from build123d import *

# Parameters (mm, degrees)
SCHIZZO1_R                   = 3.85
SCHIZZO1_R_2                 = 2.35
ESTRUSIONE_ESTRUSIONE1_DEPTH = 4
ESTRUSIONE_ESTRUSIONE2_DEPTH = 1.5
TAGLIO_ESTRUSIONE1_REACH     = 18.501
SCHIZZO4_R                   = 0.5


with BuildPart() as part:
    # Schizzo1 → Estrusione-Estrusione1 (new body)
    with BuildSketch(Plane.XY):
        Circle(SCHIZZO1_R)
        Circle(SCHIZZO1_R_2, mode=Mode.SUBTRACT)
    extrude(amount=ESTRUSIONE_ESTRUSIONE1_DEPTH)

    # Schizzo3 → Estrusione-Estrusione2 (add)
    with BuildSketch(Plane(origin=(0, 0, 0), x_dir=(-1, 0, 0), z_dir=(0, 0, -1))):
        with BuildLine():
            Line((0, 3.1), (13.85, 2))
            ThreePointArc((13.85, 2), (15.85, 0), (13.85, -2))
            Line((13.85, -2), (0, -3.1))
            ThreePointArc((0, -3.1), (-3.1, 0), (0, 3.1))
        make_face()
    extrude(amount=-ESTRUSIONE_ESTRUSIONE2_DEPTH)

    # Schizzo4 → Taglio-Estrusione1 (cut, up to next)
    with BuildSketch(Plane.XY.offset(1.5), mode=Mode.PRIVATE) as taglio_estrusione1_sk1:
        with Locations((-4.85, 0)):
            Circle(SCHIZZO4_R)
    taglio_estrusione1_tool1 = extrude(taglio_estrusione1_sk1.sketch, amount=-TAGLIO_ESTRUSIONE1_REACH, mode=Mode.PRIVATE) & part.part
    # Schizzo4 → Taglio-Estrusione1 (cut, up to next)
    with BuildSketch(Plane.XY.offset(1.5), mode=Mode.PRIVATE) as taglio_estrusione1_sk2:
        with Locations((-6.85, 0)):
            Circle(SCHIZZO4_R)
    taglio_estrusione1_tool2 = extrude(taglio_estrusione1_sk2.sketch, amount=-TAGLIO_ESTRUSIONE1_REACH, mode=Mode.PRIVATE) & part.part
    # Schizzo4 → Taglio-Estrusione1 (cut, up to next)
    with BuildSketch(Plane.XY.offset(1.5), mode=Mode.PRIVATE) as taglio_estrusione1_sk3:
        with Locations((-8.85, 0)):
            Circle(SCHIZZO4_R)
    taglio_estrusione1_tool3 = extrude(taglio_estrusione1_sk3.sketch, amount=-TAGLIO_ESTRUSIONE1_REACH, mode=Mode.PRIVATE) & part.part
    # Schizzo4 → Taglio-Estrusione1 (cut, up to next)
    with BuildSketch(Plane.XY.offset(1.5), mode=Mode.PRIVATE) as taglio_estrusione1_sk4:
        with Locations((-10.85, 0)):
            Circle(SCHIZZO4_R)
    taglio_estrusione1_tool4 = extrude(taglio_estrusione1_sk4.sketch, amount=-TAGLIO_ESTRUSIONE1_REACH, mode=Mode.PRIVATE) & part.part
    # Schizzo4 → Taglio-Estrusione1 (cut, up to next)
    with BuildSketch(Plane.XY.offset(1.5), mode=Mode.PRIVATE) as taglio_estrusione1_sk5:
        with Locations((-12.85, 0)):
            Circle(SCHIZZO4_R)
    taglio_estrusione1_tool5 = extrude(taglio_estrusione1_sk5.sketch, amount=-TAGLIO_ESTRUSIONE1_REACH, mode=Mode.PRIVATE) & part.part
    # Schizzo4 → Taglio-Estrusione1 (cut, up to next)
    with BuildSketch(Plane.XY.offset(1.5), mode=Mode.PRIVATE) as taglio_estrusione1_sk6:
        with Locations((-14.85, 0)):
            Circle(SCHIZZO4_R)
    taglio_estrusione1_tool6 = extrude(taglio_estrusione1_sk6.sketch, amount=-TAGLIO_ESTRUSIONE1_REACH, mode=Mode.PRIVATE) & part.part
    add(taglio_estrusione1_tool1.solids().sort_by_distance((-4.85, 0, 1.5))[0], mode=Mode.SUBTRACT)
    add(taglio_estrusione1_tool2.solids().sort_by_distance((-6.85, 0, 1.5))[0], mode=Mode.SUBTRACT)
    add(taglio_estrusione1_tool3.solids().sort_by_distance((-8.85, 0, 1.5))[0], mode=Mode.SUBTRACT)
    add(taglio_estrusione1_tool4.solids().sort_by_distance((-10.85, 0, 1.5))[0], mode=Mode.SUBTRACT)
    add(taglio_estrusione1_tool5.solids().sort_by_distance((-12.85, 0, 1.5))[0], mode=Mode.SUBTRACT)
    add(taglio_estrusione1_tool6.solids().sort_by_distance((-14.85, 0, 1.5))[0], mode=Mode.SUBTRACT)


solid = part.part
Could you check a few things on this model? Use its own coordinates, in mm. A direction names the side the tool comes from. Round coordinates to 2 decimals unless told otherwise and drop trailing zeros. Write each loop counter-clockwise with the first axis right and the second up, starting at its lowest first coordinate (ties: lowest second). Pieces come first, ordered by that corner, then holes. Notation, with made-up numbers: (44.5, -35.5) -> (95.5, -35.5) arc R22 ccw to (95.5, -14.5) -> close; hole circle Ø3 at (21.5, 61.25). An arc over 180 degrees is marked (long way). Use a Markdown table: item, result.
1. We'd pull the mould along Y, two halves only. Please class faces 3 (the face through (-9, -1, 1.5)), 4 (the face through (-0.509, -2.294, 2.732)), 5 (the face through (-15.85, 0.04, 0.74)): +Y half, -Y half, draft (parallel to the pull), parting line (faces both ways), or undercut.
Answer key:
| item | result |
|---|---|
| face 3 | draft |
| face 4 | undercut |
| face 5 | parting line |
2. If we section it at C-C (z = 0.7): List the corners of the cut face in (x, y) for me.
Answer key:
| item | result |
|---|---|
| outline | (-13.85, -2) -> (-2.53, -2.9) arc R3.85 ccw (long way) to (-2.53, 2.9) -> (-13.85, 2) arc R2 ccw to start; hole circle Ø1 at (-14.85, 0); hole circle Ø1 at (-12.85, 0); hole circle Ø1 at (-10.85, 0); hole circle Ø1 at (-8.85, 0); hole circle Ø1 at (-6.85, 0); hole circle Ø1 at (-4.85, 0) |
3. If we section it at B-B (x = -12.85): List the corners of the cut face in (y, z) for me.
Answer key:
| item | result |
|---|---|
| outline | (-2.08, 0) -> (-0.5, 0) -> (-0.5, 1.5) -> (-2.08, 1.5) -> close; (0.5, 0) -> (2.08, 0) -> (2.08, 1.5) -> (0.5, 1.5) -> close |
4. If we section it at A-A (y = 0): State how many separate pieces and enclosed holes the cut face has, then the cut area to 4 significant figures.
Answer key:
| item | result |
|---|---|
| separate pieces | 7 |
| enclosed holes | 0 |
| area | 28.05 mm^2 |
5. For pin 1 Ø1.5 at (x, y) = (-11, 2) entering from +Z; pin 2 Ø1 at (x, z) = (-8.5, 0.5) entering from -Y, each with a flat end and sliding along its axis, tell me the tip position at first contact or that it passes through.
Answer key:
| item | result |
|---|---|
| pin 1 | stops at z = 1.5 |
| pin 2 | stops at y = -2.46 |
6. Which directions (+Z, -Z, +X, -X, +Y, -Y) give clear straight access to the entire face, cutting with the end or side of a thin tool? Please do faces 1 (the face through (0, 0, 1.5)), 2 (the face through (-4, 0, 0)).
Answer key:
| item | result |
|---|---|
| face 1 | +Z |
| face 2 | -Z, +X, -X, +Y, -Y |
7. Please list where these lines run through material, in increasing order: probe 1 along Y at (x, z) = (0, 3.45); probe 2 along Y at (x, z) = (-9.5, 0.25).
Answer key:
| item | result |
|---|---|
| probe 1 | y = -3.85 to -2.35, 2.35 to 3.85 |
| probe 2 | y = -2.35 to 2.35 |
8. If we section it at D-D (z = 3.15): List the corners of the cut face in (x, y) for me, then the cut area to 3 significant figures.
Answer key:
| item | result |
|---|---|
| outline | circle Ø7.7 at (0, 0); hole circle Ø4.7 at (0, 0) |
| area | 29.2 mm^2 |
